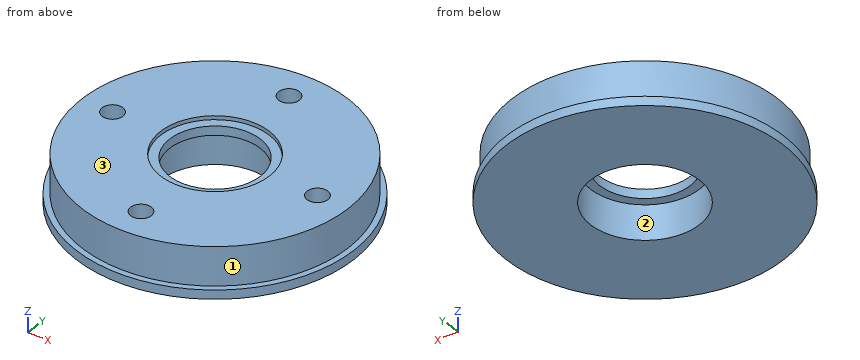
```python
from build123d import *

# Parameters (mm, degrees)
SKETCH1_R           = 30.625
SKETCH1_R_2         = 29.375
SKETCH1_R_3         = 12
BOSS_EXTRUDE1_DEPTH = 2
BOSS_EXTRUDE2_START = 2
SKETCH1_3_R         = 29.375
SKETCH1_3_R_2       = 12
BOSS_EXTRUDE2_DEPTH = 8.5
BOSS_EXTRUDE3_START = 7.65
SKETCH1_4_R         = 12
SKETCH1_4_R_2       = 10
BOSS_EXTRUDE3_DEPTH = 2
SKETCH2_R           = 2.3
CUT_EXTRUDE1_DEPTH  = 9


with BuildPart() as part:
    # Sketch1 → Boss-Extrude1 (new body)
    # profile 1 of 2: a face of its own
    with BuildSketch(Plane.XY):
        Circle(SKETCH1_R)
        Circle(SKETCH1_R_2, mode=Mode.SUBTRACT)
    # profile 2 of 2: a face of its own
    with BuildSketch(Plane.XY):
        Circle(SKETCH1_R_2)
        Circle(SKETCH1_R_3, mode=Mode.SUBTRACT)
    extrude(amount=BOSS_EXTRUDE1_DEPTH)

    # Sketch1<3> → Boss-Extrude2 (add)
    with BuildSketch(Plane.XY.offset(BOSS_EXTRUDE2_START)):
        Circle(SKETCH1_3_R)
        Circle(SKETCH1_3_R_2, mode=Mode.SUBTRACT)
    extrude(amount=BOSS_EXTRUDE2_DEPTH)

    # Sketch1<4> → Boss-Extrude3 (add)
    with BuildSketch(Plane.XY.offset(BOSS_EXTRUDE3_START)):
        Circle(SKETCH1_4_R)
        Circle(SKETCH1_4_R_2, mode=Mode.SUBTRACT)
    extrude(amount=BOSS_EXTRUDE3_DEPTH)

    # Sketch2 → Cut-Extrude1 (cut)
    with BuildSketch(Plane.XY.offset(10.5)):
        with Locations((0, 22.5)):
            Circle(SKETCH2_R)
        with Locations((22.5, 0)):
            Circle(SKETCH2_R)
        with Locations((0, -22.5)):
            Circle(SKETCH2_R)
        with Locations((-22.5, 0)):
            Circle(SKETCH2_R)
    extrude(amount=-CUT_EXTRUDE1_DEPTH, mode=Mode.SUBTRACT)


solid = part.part
```
Check sheet for the modelled part. Datum: model origin and axes. Units: mm. Face numbers are marked on the shaded views. Coordinates: 2 decimals unless noted, no trailing zeros. Order: outer loops, then holes, each group sorted by start corner. A loop starts at its lowest first (then second) coordinate and runs counter-clockwise, first axis right, second up. Notation, with made-up numbers: M 67.5,-36.5 L 125.5,-36.5 A11 cw 125.5,-19.5 Z; hole C -14.5,61.5 d1. An arc over 180 degrees is marked long. Write each question's results on one line, items separated by ' | '. Start each with the question number.
1. Cross-section at B-B on y = -7. Record the cut outline in (x, z).
2. Go/stop test with flat-tipped pins: P1, Ø4, axis at x = 4, z = 8.5, coming from the -Y side; P2, Ø6, axis at y = 10, z = 2.5, coming from the -X side; P3, Ø2, axis at y = 7, z = 6.5, coming from the +X side. Record where each tip stops, or that it passes through.
3. Cross-section at D-D on y = -17. Record the cut outline in (x, z), and give its area (3 significant figures).
4. Cross-section at C-C on x = 8.5. Record the cut outline in (y, z), and give its area (3 significant figures).
5. Material ranges on probe 1 along Y at (x, z) = (0, 10.1) (3 decimals); probe 2 along Y at (x, z) = (-1, 9.75); probe 3 along Z at (x, y) = (4.5, -9.5), recorded low to high.
6. Cross-section at A-A on z = 3. Record the cut outline in (x, y) (3 decimals), and give its area (3 significant figures).
7. Mould release check, pull along X, two halves, no side actions. Record for the marked faces 1, 2 and 3: +X half, -X half, draft (parallel to the pull), parting line (faces both ways), or undercut.
Checks:
1) outline: M -29.81,0 L -9.75,0 L -9.75,7.65 L -7.14,7.65 L -7.14,9.65 L -9.75,9.65 L -9.75,10.5 L -28.53,10.5 L -28.53,2 L -29.81,2 Z; M 7.14,7.65 L 9.75,7.65 L 9.75,0 L 29.81,0 L 29.81,2 L 28.53,2 L 28.53,10.5 L 9.75,10.5 L 9.75,9.65 L 7.14,9.65 Z
2) P1: stops at y = -29.31 | P2: stops at x = -29.8 | P3: stops at x = 28.76
3) outline: M -25.47,0 L 25.47,0 L 25.47,2 L 23.96,2 L 23.96,10.5 L -23.96,10.5 L -23.96,2 L -25.47,2 Z | area: 509 mm²
4) outline: M -29.42,0 L -8.47,0 L -8.47,7.65 L -5.27,7.65 L -5.27,9.65 L -8.47,9.65 L -8.47,10.5 L -28.12,10.5 L -28.12,2 L -29.42,2 Z; M 5.27,7.65 L 8.47,7.65 L 8.47,0 L 29.42,0 L 29.42,2 L 28.12,2 L 28.12,10.5 L 8.47,10.5 L 8.47,9.65 L 5.27,9.65 Z | area: 431 mm²
5) probe 1: y = -29.375 to -24.8, -20.2 to -12, 12 to 20.2, 24.8 to 29.375 | probe 2: y = -29.36 to -24.57, -20.43 to -11.96, 11.96 to 20.43, 24.57 to 29.36 | probe 3: z = 7.65 to 9.65
6) outline: C 0,0 d58.75; hole C -22.5,0 d4.6; hole C 0,0 d24; hole C 0,-22.5 d4.6; hole C 0,22.5 d4.6; hole C 22.5,0 d4.6 | area: 2,190 mm²
7) face 1: parting line | face 2: undercut | face 3: draft
